Can you work these out from the drawing? Everything is in mm from the part's minimum corner. A direction names the side the tool comes from. Round coordinates to 2 decimals unless told otherwise and drop trailing zeros. Write each loop counter-clockwise with the first axis right and the second up, starting at its lowest first coordinate (ties: lowest second). Pieces come first, ordered by that corner, then holes.
Q1. For the marked faces 4, 5 and 6, which set-ups out of +Z, -Z, +X, -X, +Y, -Y let a thin tool reach every point of the face, with its end or its side?
Q2. We'd pull the mould along Z, two halves only. Please class the marked faces 1, 2 and 3: +Z half, -Z half, draft (parallel to the pull), parting line (faces both ways), or undercut.
Q3. I'm going to push flat-ended pins straight in: pin 1 Ø8 at (y, z) = (7, 4) entering from -X; pin 2 Ø2.5 at (x, z) = (8, 7) entering from +Y (1 decimal); pin 3 Ø5 at (y, z) = (11.5, 2.5) entering from -X. Where does each tip first touch, or does it pass through?
Q4. If we section it at C-C (y = 6.75): Please give me the cut outline in (x, z).
Q5. If we section it at D-D (z = 3.25): Please give me the cut outline in (x, y), plus the area to 3 significant figures.
Q6. Please list where these lines run through material, in increasing order: line 1 along Z through (x, y) = (8, 19.5) (1 decimal); line 2 along Y through (x, z) = (8.75, 8) (1 decimal); line 3 along Y through (x, z) = (10, 15.25).
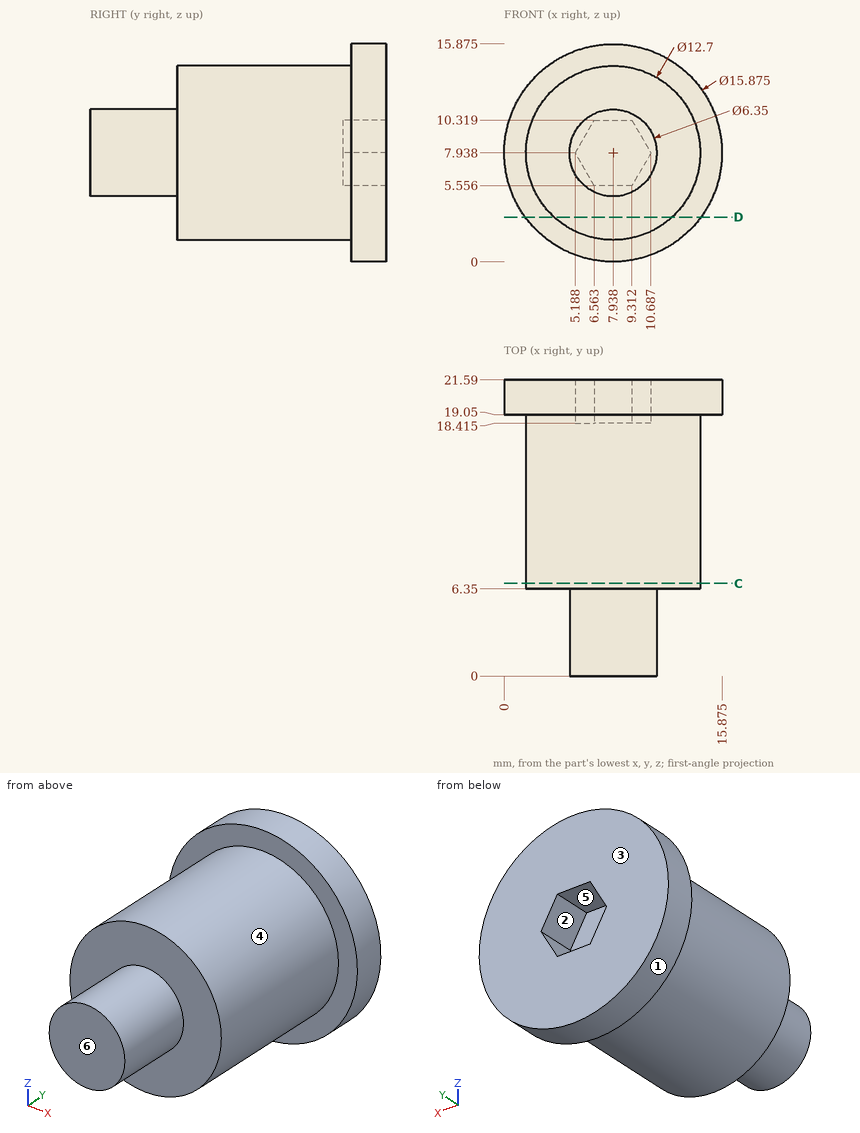
A:
1. face 4: -Y
1. face 5: +Y
1. face 6: +Z, -Z, +X, -X, -Y
2. face 1: parting line
2. face 2: undercut
2. face 3: draft
3. pin 1: stops at x = 1.59
3. pin 2: stops at y = 18.4
3. pin 3: stops at x = 2.31
4. outline: circle Ø12.7 at (7.94, 7.94)
5. outline: (1.53, 19.05) - (3.65, 19.05) - (3.65, 6.35) - (12.22, 6.35) - (12.22, 19.05) - (14.34, 19.05) - (14.34, 21.59) - (1.53, 21.59) - close
5. area: 141 mm2
6. line 1: z = 0 to 5.6, 10.3 to 15.9
6. line 2: y = 0 to 18.4
6. line 3: y = 19.05 to 21.59
